Can you work these out from the model? Positions are in its coordinate system, mm. A direction names the side the tool comes from. Give positions to 0.01 mm unless a question says otherwise; leave off trailing zeros. Loops run counter-clockwise (first coordinate to the right, second up) from the corner with the lowest first, then second, coordinate; pieces in that order, holes last. Notation, with made-up numbers: (-11.75, 39) - (-0.75, 39) arc R9 ccw to (-0.75, 44) - close; hole circle Ø3 at (59.25, -29.5). An arc over 180 degrees is marked (long way). Answer as a JSON object with one key per item and string values.
```python
from build123d import *

# Parameters (mm, degrees)
SKETCH1_W           = 600
SKETCH1_H           = 120
BOSS_EXTRUDE1_DEPTH = 20
CUT_EXTRUDE1_REACH  = 325.728
SKETCH6_W           = 500
SKETCH6_H           = 25
SKETCH6_H_2         = 45
CUT_EXTRUDE2_DEPTH  = 12.7
FILLET1_R           = 10
FILLET2_R           = 5
CUT_EXTRUDE3_REACH  = 308.594
SKETCH7_W           = 50
SKETCH7_H           = 100


with BuildPart() as part:
    # Sketch1 → Boss-Extrude1 (new body)
    with BuildSketch(Plane(origin=(0, 0, 0), x_dir=(1, 0, 0), z_dir=(0, 1, 0))):
        Rectangle(SKETCH1_W, SKETCH1_H)
    extrude(amount=BOSS_EXTRUDE1_DEPTH)

    # Sketch4 → Cut-Extrude1 (cut, up to next)
    with BuildSketch(Plane.XY.offset(60), mode=Mode.PRIVATE) as cut_extrude1_sk1:
        Polygon((-300, 10), (-250, 0), (-300, 0), align=None)
    cut_extrude1_tool1 = extrude(cut_extrude1_sk1.sketch, amount=-CUT_EXTRUDE1_REACH, mode=Mode.PRIVATE) & part.part
    add(cut_extrude1_tool1.solids().sort_by_distance((-283.333333, 3.333333, 60))[0], mode=Mode.SUBTRACT)

    # Sketch6 → Cut-Extrude2 (cut)
    with BuildSketch(Plane(origin=(0, 20, 0), x_dir=(1, 0, 0), z_dir=(0, 1, 0))):
        with Locations((30, 27.5)):
            Rectangle(SKETCH6_W, SKETCH6_H)
        with Locations((30, -17.5)):
            Rectangle(SKETCH6_W, SKETCH6_H_2)
    extrude(amount=-CUT_EXTRUDE2_DEPTH, mode=Mode.SUBTRACT)

    # Fillet1
    fillet1_edges = [part.edges().sort_by_distance(p)[0] for p in [
        (-300, 15, -60),
        (300, 10, -60),
        (300, 10, 60),
        (-300, 15, 60),
    ]]
    fillet(fillet1_edges, radius=FILLET1_R)

    # Fillet2
    fillet2_edges = [part.edges().sort_by_distance(p)[0] for p in [
        (-220, 13.65, -15),
        (-220, 13.65, -40),
        (280, 13.65, -40),
        (280, 13.65, -15),
    ]]
    fillet(fillet2_edges, radius=FILLET2_R)

    # Sketch7 → Cut-Extrude3 (cut, up to next)
    with BuildSketch(Plane(origin=(0, 20, 0), x_dir=(1, 0, 0), z_dir=(0, 1, 0)), mode=Mode.PRIVATE) as cut_extrude3_sk1:
        with Locations((-275, 0)):
            Rectangle(SKETCH7_W, SKETCH7_H)
    cut_extrude3_tool1 = extrude(cut_extrude3_sk1.sketch, amount=-CUT_EXTRUDE3_REACH, mode=Mode.PRIVATE) & part.part
    add(cut_extrude3_tool1.solids().sort_by_distance((-275, 20, 0))[0], mode=Mode.SUBTRACT)


solid = part.part
```
1) Imagine slicing it at C-C on z = 18. Write out the boundary of the cut face in (x, y).
Check sheet entries:
{"outline": "(-250, 0) - (300, 0) - (300, 20) - (280, 20) - (280, 7.3) - (-220, 7.3) - (-220, 20) - (-250, 20) - close"}
2) I need wall thicknesses on L1, parallel to Z at x = -170, y = 18; L2, parallel to X at y = 9, z = 23; L3, parallel to Y at x = -199.5, z = 33. Which ranges of each line are inside material? Lowest first, please.
Check sheet entries:
{"L1": "-60 to -40, -15 to -5, 40 to 60", "L2": "-250 to -220, 280 to 300", "L3": "0 to 7.3"}
3) I'm going to push flat-ended pins straight in: P1, Ø2, axis at x = 72.5, z = 11.5, coming from the +Y side; P2, Ø6.5, axis at y = 14, z = -29, coming from the -X side. Where does each tip first touch, or does it pass through?
Check sheet entries:
{"P1": "y = 7.3", "P2": "x = -250"}
4) Which directions (+Z, -Z, +X, -X, +Y, -Y) give clear straight access to the entire face, cutting with the end or side of a thin tool? Please do faces 1 (the cylindrical face through (296.99, 10.14, 57.15)), 2 (the flat face through (-275, 12, 50)), 3 (the flat face through (27, 14, 40)).
Check sheet entries:
{"face 1": "+Z, +X, +Y, -Y", "face 2": "-X, +Y, -Y", "face 3": "+Y"}
5) If we mould it in two halves opening along Z, with no side actions, what happens to faces 4 (the flat face through (-220, 14, 18)), 5 (the cylindrical face through (296.99, 10.14, -57.15)), 6 (the flat face through (-275, 5, -55))? For each: released by +Z, released by -Z, zero draft, split by the parting line, or undercut.
Check sheet entries:
{"face 4": "undercut", "face 5": "released by -Z", "face 6": "zero draft"}
6) Imagine slicing it at A-A on y = 14. Write out the boundary of the cut face in (x, z).
Check sheet entries:
{"outline": "(-300, -50) arc R10 ccw to (-290, -60) - (290, -60) arc R10 ccw to (300, -50) - (300, 50) arc R10 ccw to (290, 60) - (-290, 60) arc R10 ccw to (-300, 50) - (-250, 50) - (-250, -50) - close; hole (-220, -35) arc R5 ccw to (-215, -40) - (275, -40) arc R5 ccw to (280, -35) - (280, -20) arc R5 ccw to (275, -15) - (-215, -15) arc R5 ccw to (-220, -20) - close; hole (-220, -5) - (280, -5) - (280, 40) - (-220, 40) - close"}
7) Imagine slicing it at B-B on x = 37.5. Write out the boundary of the cut face in (y, z), and give its area (3 significant figures).
Check sheet entries:
{"outline": "(0, -60) - (20, -60) - (20, -40) - (7.3, -40) - (7.3, -15) - (20, -15) - (20, -5) - (7.3, -5) - (7.3, 40) - (20, 40) - (20, 60) - (0, 60) - close", "area": "1,510 mm2"}
